```python
from build123d import *

# Parameters (mm, degrees)
SKETCH1_R           = 21.59
BOSS_EXTRUDE1_DEPTH = 6.35
SKETCH2_R           = 15.875
BOSS_EXTRUDE2_DEPTH = 50.8
FILLET1_R           = 2.54
SKETCH3_R           = 21.59
BOSS_EXTRUDE3_DEPTH = 6.35
FILLET2_R           = 2.54
SKETCH4_R           = 4.7625
CUT_EXTRUDE1_DEPTH  = 71.459252054


with BuildPart() as part:
    # Sketch1 → Boss-Extrude1 (new body)
    with BuildSketch(Plane(origin=(0, 0, 0), x_dir=(0, 0, -1), z_dir=(1, 0, 0))):
        Circle(SKETCH1_R)
    extrude(amount=BOSS_EXTRUDE1_DEPTH)

    # Sketch2 → Boss-Extrude2 (add)
    with BuildSketch(Plane(origin=(6.35, 0, 0), x_dir=(0, 0, -1), z_dir=(1, 0, 0))):
        Circle(SKETCH2_R)
    extrude(amount=BOSS_EXTRUDE2_DEPTH)

    # Fillet1
    fillet1_edges = [part.edges().sort_by_distance(p)[0] for p in [
        (6.35, 0, 15.875),
    ]]
    fillet(fillet1_edges, radius=FILLET1_R)

    # Sketch3 → Boss-Extrude3 (add)
    with BuildSketch(Plane(origin=(57.15, 0, 0), x_dir=(0, 0, -1), z_dir=(1, 0, 0))):
        Circle(SKETCH3_R)
    extrude(amount=BOSS_EXTRUDE3_DEPTH)

    # Fillet2
    fillet2_edges = [part.edges().sort_by_distance(p)[0] for p in [
        (57.15, 0, 15.875),
    ]]
    fillet(fillet2_edges, radius=FILLET2_R)

    # Sketch4 → Cut-Extrude1 (cut, through all)
    with BuildSketch(Plane(origin=(63.5, 0, 0), x_dir=(0, 0, -1), z_dir=(1, 0, 0))):
        Circle(SKETCH4_R)
    extrude(amount=-CUT_EXTRUDE1_DEPTH, mode=Mode.SUBTRACT)


solid = part.part
```
Check sheet for the modelled part. Datum: model origin and axes. Units: mm. A direction names the side the tool comes from. Give positions to 0.01 mm unless a question says otherwise; leave off trailing zeros. Write each loop counter-clockwise with the first axis right and the second up, starting at its lowest first coordinate (ties: lowest second). Pieces come first, ordered by that corner, then holes. Notation, with made-up numbers: (43.5, 6) - (90.5, 6) arc R22 cw to (90.5, 25) - close; hole circle Ø6 at (57.5, 28). An arc over 180 degrees is marked (long way). Answer as a JSON object with one key per item and string values. Group by question number.
1) Sectioned sample at D-D (x = 4.5). Record the cut outline in (y, z) (1 decimal), then the cut area to 3 significant figures.
2) Access from +Z, -Z, +X, -X, +Y, -Y to the whole of each face (thin tool, end or side, straight path). Record for faces 4 (the face through (32.19, -2.9, 3.78)), 5 (the face through (6.35, 10, -16)).
3) Depth check by flat-ended pin: P1, Ø1, axis at x = 37.5, y = -6, coming from the -Z side; P2, Ø6, axis at x = 45.5, z = 0, coming from the -Y side (3 decimals); P3, Ø12, axis at x = 18, z = 13.5, coming from the +Y side; P4, Ø15, axis at y = 0, z = 0, coming from the +X side. Enter the tip coordinate at first touch or a pass-through.
4) Thickness scan on probe 1 along X at (y, z) = (11, 18.5); probe 2 along Y at (x, z) = (45.5, 0) (1 decimal); probe 3 along Y at (x, z) = (28, 3). Record the ranges inside material, lowest first. Write a range as from..to.
5) Release check for a two-part mould opening along X. For faces 1 (the face through (63.5, 5, 0)), 2 (the face through (57.15, 10, -16)), 3 (the face through (3.131, 14.592, 15.913)) record: pulls with the +X half, pulls with the -X half, needs draft (parallel to the pull), parting line crosses it, or undercut.
Geometry results:
{
 "1": {"outline": "circle Ø43.2 at (0, 0); hole circle Ø9.5 at (0, 0)", "area": "1,390 mm^2"},
 "2": {"face 4": "+X, -X", "face 5": "none"},
 "3": {"P1": "stops at z = -14.89", "P2": "stops at y = -15.875", "P3": "stops at y = 13.99", "P4": "stops at x = 63.5"},
 "4": {"probe 1": "x = 0..6.35, 57.15..63.5", "probe 2": "y = -15.9..-4.8, 4.8..15.9", "probe 3": "y = -15.59..-3.7, 3.7..15.59"},
 "5": {"face 1": "pulls with the +X half", "face 2": "undercut", "face 3": "needs draft"}
}
